Autodesk Inventor part; units mm, degrees
ref_plane "YZ Plane" through (0, 0, 0) normal (1, 0, 0) x (0, 1, 0)
ref_plane "XZ Plane" through (0, 0, 0) normal (0, 1, 0) x (-1, 0, 0)
ref_plane "XY Plane" through (0, 0, 0) normal (0, 0, 1) x (1, 0, 0)
sketch "Sketch1" plane through (0, 0, 0) normal (0, 0, 1) x (1, 0, 0)
  line L0 (-30.2941, 0) -> (30.2941, 0)
  line L1 (-14.605, 12.7) -> (14.605, 12.7)
  line L2 (14.605, 12.7) -> (14.605, 16.002)
  line L3 (14.605, 16.002) -> (6.985, 16.002)
  line L4 (6.985, 16.002) -> (6.985, 14.478)
  line L5 (6.985, 14.478) -> (4.445, 14.478)
  line L6 (4.445, 14.478) -> (4.445, 19.05)
  line L7 (4.445, 19.05) -> (-20.955, 19.05)
  line L8 (-20.955, 19.05) -> (-20.955, 9.525)
  line L9 (-20.955, 9.525) -> (-14.605, 9.525)
  line L10 (-14.605, 9.525) -> (-14.605, 12.7)
  point P0 (0, 0)
  point P1 (0, 0)
  point P2 (0, 12.7)
  dimension "d0" = 25.4
  dimension "d2" = 19.05
  dimension "d3" = 6.35
  dimension "d4" = 38.1
  dimension "d6" = 19.05
  dimension "d7" = 32.004
  dimension "d8" = 1.524
  dimension "d16" = 10.16
  dimension "d17" = 2.54
revolve "Revolution1" add sketch "Sketch1" angle 360 about axis through (-30.2941, 0, 0) along (1, 0, 0)
thread "Thread1"
chamfer "Chamfer1" distance 0.7937 angle 45 5 edges at (14.605, -16.002, 0) (14.605, -12.7, 0) (-14.605, -9.525, 0) (-20.955, -9.525, 0) (-20.955, -19.05, 0)
properties part number "PommelPart" material "Aluminum 6061"
For this review, take the finished solid that the model builds, in its own axes (mm). A direction names the side the tool comes from. Round coordinates to 2 decimals unless told otherwise and drop trailing zeros. Loops run counter-clockwise (first coordinate to the right, second up) from the corner with the lowest first, then second, coordinate; pieces in that order, holes last. Notation, with made-up numbers: (87.25, 12.25) - (131.25, 12.25) arc R10 cw to (131.25, 18.25) - close; hole circle Ø1 at (25.5, 51). An arc over 180 degrees is marked (long way). Use one line per item in the form item = value.
1) Clearance check with flat-ended pins moving along their axes: P1, Ø1, axis at x = -5, z = 8.5, coming from the -Y side; P2, Ø1, axis at x = -9.5, z = 10, coming from the -Y side; P3, Ø8, axis at x = -17, z = 9, coming from the +Y side; P4, Ø9.5, axis at y = -5, z = -3, coming from the -X side (3 decimals). State where each tip first meets the part, or that it passes through.
Solutions:
P1 = -17.29
P2 = -16.51
P3 = 18.38
P4 = -20.955
2) Wall thickness on probe 1 along Z at (x, y) = (-17.5, 0) (3 decimals); probe 2 along Z at (x, y) = (-3, 0); probe 3 along X at (y, z) = (14.5, 3) (3 decimals): over which ranges is each line inside the solid? List them lowest first.
Solutions:
probe_1 = -19.05 to -9.525, 9.525 to 19.05
probe_2 = -19.05 to -12.7, 12.7 to 19.05
probe_3 = -20.955 to 4.445, 6.985 to 14.605
3) We need section C-C on x = 2.5. Write out the cut boundary in (y, z), then the cut area to 3 significant figures.
Solutions:
outline = circle Ø38.1 at (0, 0); hole circle Ø25.4 at (0, 0)
area = 633 mm2
4) Mouldability with a two-part tool opening along Y and no side actions: class faces 1 (the face through (-17.747, -7.559, -5.796)), 2 (the face through (5.697, -1.885, -14.355)), 3 (the face through (-20.955, 8, -8)), 4 (the face through (-14.605, -1.9, 10.4)) as pulls with the +Y half, pulls with the -Y half, needs draft (parallel to the pull), parting line crosses it, or undercut.
Solutions:
face_1 = undercut
face_2 = parting line crosses it
face_3 = needs draft
face_4 = undercut
5) Tool access review of faces 5 (the face through (10.35, -3.47, 15.62)), 6 (the face through (14.605, -2.32, -13.45)), 7 (the face through (4.445, 13, 7)): name each direction out of +Z, -Z, +X, -X, +Y, -Y from which nothing blocks a thin tool from reaching the whole face with its end or side.
Solutions:
face_5 = +X
face_6 = +Z, -Z, +X, +Y, -Y
face_7 = none
